Answer from the drawing. Dimensions are ordinates in mm from the lowest x, y and z of the part. A direction names the side the tool comes from. Give positions to 0.01 mm unless a question says otherwise; leave off trailing zeros. Order: outer loops, then holes, each group sorted by start corner. A loop starts at its lowest first (then second) coordinate and runs counter-clockwise, first axis right, second up. Notation, with made-up numbers: (86, 89) - (104, 89) arc R6 ccw to (104, 98) - close; hole circle Ø11 at (-9, 22). An arc over 180 degrees is marked (long way). Answer in a Markdown table with one row per item. Add a question column.
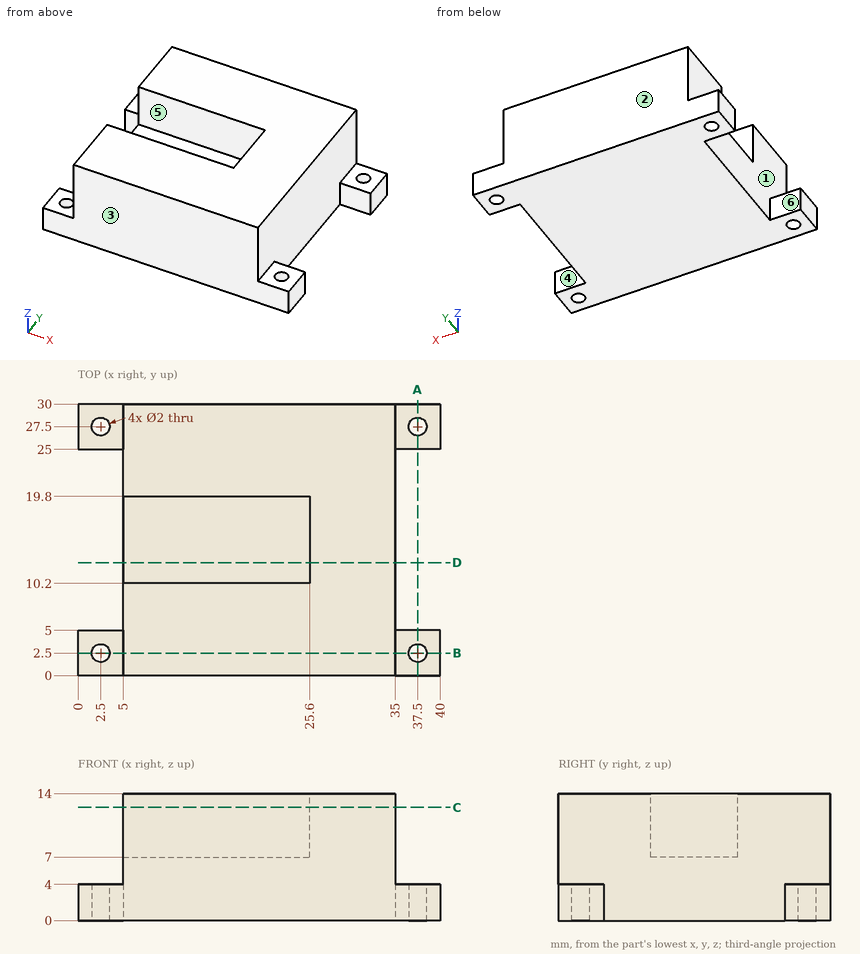
(1) Find section B-B, the plane y = 2.5. Write down the section's boundary in (x, z), plus the area to 3 significant figures.
(2) For the marked faces 4, 5 and 6, determine the directions among +Z, -Z, +X, -X, +Y, -Y from which every point of the face is accessible in a straight line to the end or side of a thin tool.
(3) Find section A-A, the plane x = 37.5. Write down the section's boundary in (y, z).
(4) Straight lines are drawn through the part: line 1 (Y direction, x = 2.5, z = 0.9); line 2 (Y direction, x = 21, z = 9.5); line 3 (X direction, y = 13.5, z = 8.25). For each, find the intervals that lie inside material, in ascending order.
(5) Find section D-D, the plane y = 12.5. Write down the section's boundary in (x, z).
(6) Each of these flat-tipped pins is pushed along its axis until it touches: P1, Ø2, axis at y = 14, z = 9.5, coming from the -X side; P2, Ø1.8, axis at x = 37.5, y = 2.5, coming from the -Z side; P3, Ø3, axis at x = 37.5, y = 27.5, coming from the +Z side; P4, Ø3, axis at y = 9, z = 11, coming from the +X side. Where does it stop, or does it pass through?
(7) The mould has two halves that part along Y. Classify the marked faces 1, 2 and 3: +Y half, -Y half, draft (parallel to the pull), parting line (faces both ways), or undercut.
(8) Find section C-C, the plane z = 12.5. Write down the section's boundary in (x, y).
Answer key:
| question | item | result |
|---|---|---|
| 1 | outline | (0, 0) - (1.5, 0) - (1.5, 4) - (0, 4) - close; (3.5, 0) - (36.5, 0) - (36.5, 4) - (35, 4) - (35, 14) - (5, 14) - (5, 4) - (3.5, 4) - close; (38.5, 0) - (40, 0) - (40, 4) - (38.5, 4) - close |
| 1 | area | 444 mm² |
| 2 | face 4 | +Z, -Z, +X |
| 2 | face 5 | +Z, -X |
| 2 | face 6 | +Z, -Z, -X |
| 3 | outline | (0, 0) - (1.5, 0) - (1.5, 4) - (0, 4) - close; (3.5, 0) - (5, 0) - (5, 4) - (3.5, 4) - close; (25, 0) - (26.5, 0) - (26.5, 4) - (25, 4) - close; (28.5, 0) - (30, 0) - (30, 4) - (28.5, 4) - close |
| 4 | line 1 | 0 to 1.5, 3.5 to 5, 25 to 26.5, 28.5 to 30 |
| 4 | line 2 | 0 to 10.2, 19.8 to 30 |
| 4 | line 3 | 25.6 to 35 |
| 5 | outline | (5, 0) - (35, 0) - (35, 14) - (25.6, 14) - (25.6, 7) - (5, 7) - close |
| 6 | P1 | x = 25.6 |
| 6 | P2 | through |
| 6 | P3 | z = 4 |
| 6 | P4 | x = 35 |
| 7 | face 1 | undercut |
| 7 | face 2 | +Y half |
| 7 | face 3 | -Y half |
| 8 | outline | (5, 0) - (35, 0) - (35, 30) - (5, 30) - (5, 19.8) - (25.6, 19.8) - (25.6, 10.2) - (5, 10.2) - close |
